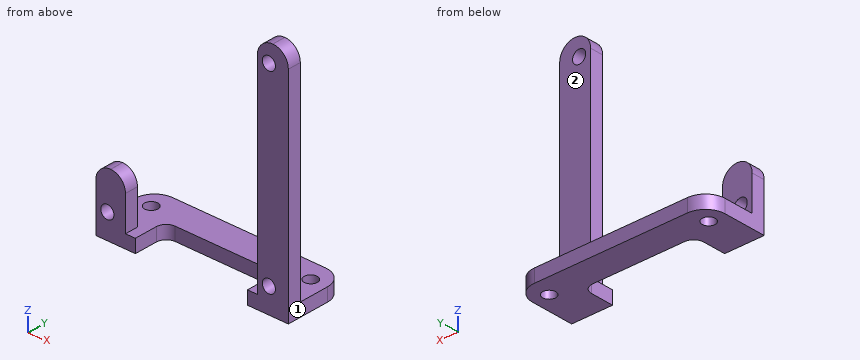
```python
from build123d import *

# Parameters (mm, degrees)
CYLINDER393_R     = 2
CYLINDER393_DEPTH = 16
CYLINDER395_R     = 2
CYLINDER395_DEPTH = 16
CYLINDER394_R     = 2
CYLINDER394_DEPTH = 16
BOX490_W          = 34
BOX490_H          = 10
BOX490_DEPTH      = 7
FILLET028_R       = 3
BOX489_W          = 58.4
BOX489_H          = 19
BOX489_DEPTH      = 4
FILLET029_R       = 6
CYLINDER384_R     = 2
CYLINDER384_DEPTH = 10
CYLINDER385_R     = 2
CYLINDER385_DEPTH = 10
BOX482_W          = 9.4
BOX482_H          = 4
BOX482_DEPTH      = 67
FILLET025_R       = 4.69
CYLINDER386_R     = 2
CYLINDER386_DEPTH = 10
BOX480_W          = 9
BOX480_H          = 4
BOX480_DEPTH      = 15
FILLET024_R       = 4.49


with BuildPart() as cylinder393:
    # Cylinder393 → Cylinder393 (new body)
    with BuildSketch(Plane(origin=(-9.8, 51, -5), x_dir=(1, 0, 0), z_dir=(0, 0, 1))):
        Circle(CYLINDER393_R)
    extrude(amount=CYLINDER393_DEPTH)


with BuildPart() as cylinder395:
    # Cylinder395 → Cylinder395 (new body)
    with BuildSketch(Plane(origin=(-58.2, 51, -5), x_dir=(1, 0, 0), z_dir=(0, 0, 1))):
        Circle(CYLINDER395_R)
    extrude(amount=CYLINDER395_DEPTH)


with BuildPart() as fusion386:
    # Cylinder394 → Cylinder394 (new body)
    with BuildSketch(Plane(origin=(-9.8, 51, -5), x_dir=(1, 0, 0), z_dir=(0, 0, 1))):
        Circle(CYLINDER394_R)
    extrude(amount=CYLINDER394_DEPTH)

    # Fusion386: union Cylinder393, Cylinder395
    add(cylinder393.part)
    add(cylinder395.part)


with BuildPart() as fillet028:
    # Box490 → Box490 (new body)
    with BuildSketch(Plane(origin=(-51.2, 38, 0), x_dir=(1, 0, 0), z_dir=(0, 0, 1))):
        with Locations((17, 5)):
            Rectangle(BOX490_W, BOX490_H)
    extrude(amount=BOX490_DEPTH)

    # Fillet028
    fillet028_edges = [fillet028.edges().sort_by_distance(p)[0] for p in [
        (-51.2, 48, 3.5),
        (-17.2, 48, 3.5),
    ]]
    fillet(fillet028_edges, radius=FILLET028_R)


with BuildPart() as fillet029:
    # Box489 → Box489 (new body)
    with BuildSketch(Plane(origin=(-63.2, 38, 3), x_dir=(1, 0, 0), z_dir=(0, 0, 1))):
        with Locations((29.2, 9.5)):
            Rectangle(BOX489_W, BOX489_H)
    extrude(amount=BOX489_DEPTH)

    # Cut421: cut Fillet028
    add(fillet028.part, mode=Mode.SUBTRACT)

    # Cut422: cut Fusion386
    add(fusion386.part, mode=Mode.SUBTRACT)

    # Fillet029
    fillet029_edges = [fillet029.edges().sort_by_distance(p)[0] for p in [
        (-63.2, 57, 5),
        (-4.8, 57, 5),
    ]]
    fillet(fillet029_edges, radius=FILLET029_R)


with BuildPart() as cylinder384:
    # Cylinder384 → Cylinder384 (new body)
    with BuildSketch(Plane(origin=(-10.7, 44, 10.5), x_dir=(1, 0, 0), z_dir=(0, -1, 0))):
        Circle(CYLINDER384_R)
    extrude(amount=CYLINDER384_DEPTH)


with BuildPart() as fusion379:
    # Cylinder385 → Cylinder385 (new body)
    with BuildSketch(Plane(origin=(-10.7, 44, 68.5), x_dir=(1, 0, 0), z_dir=(0, -1, 0))):
        Circle(CYLINDER385_R)
    extrude(amount=CYLINDER385_DEPTH)

    # Fusion379: union Cylinder384
    add(cylinder384.part)


with BuildPart() as fillet025:
    # Box482 → Box482 (new body)
    with BuildSketch(Plane(origin=(-14.2, 38, 7), x_dir=(1, 0, 0), z_dir=(0, 0, 1))):
        with Locations((4.7, 2)):
            Rectangle(BOX482_W, BOX482_H)
    extrude(amount=BOX482_DEPTH)

    # Cut417: cut Fusion379
    add(fusion379.part, mode=Mode.SUBTRACT)

    # Fillet025
    fillet025_edges = [fillet025.edges().sort_by_distance(p)[0] for p in [
        (-14.2, 40, 74),
        (-4.8, 40, 74),
    ]]
    fillet(fillet025_edges, radius=FILLET025_R)


with BuildPart() as cylinder386:
    # Cylinder386 → Cylinder386 (new body)
    with BuildSketch(Plane(origin=(-59.7, 44, 10.5), x_dir=(1, 0, 0), z_dir=(0, -1, 0))):
        Circle(CYLINDER386_R)
    extrude(amount=CYLINDER386_DEPTH)


with BuildPart() as fusion388:
    # Box480 → Box480 (new body)
    with BuildSketch(Plane(origin=(-63.2, 38, 7), x_dir=(1, 0, 0), z_dir=(0, 0, 1))):
        with Locations((4.5, 2)):
            Rectangle(BOX480_W, BOX480_H)
    extrude(amount=BOX480_DEPTH)

    # Cut418: cut Cylinder386
    add(cylinder386.part, mode=Mode.SUBTRACT)

    # Fillet024
    fillet024_edges = [fusion388.edges().sort_by_distance(p)[0] for p in [
        (-63.2, 40, 22),
        (-54.2, 40, 22),
    ]]
    fillet(fillet024_edges, radius=FILLET024_R)

    # Fusion388: union Fillet029, Fillet025
    add(fillet029.part)
    add(fillet025.part)


solid = fusion388.part
```
The listing builds one solid part. Answer for the finished solid, in the listing's coordinates (mm). Face numbers are marked on the shaded views. A direction names the side the tool comes from. Round coordinates to 2 decimals unless told otherwise and drop trailing zeros. Loops run counter-clockwise (first coordinate to the right, second up) from the corner with the lowest first, then second, coordinate; pieces in that order, holes last. Notation, with made-up numbers: (32, 41.5) - (84, 41.5) arc R19 cw to (84, 64.5) - close; hole circle Ø1 at (57.5, 44). An arc over 180 degrees is marked (long way). Use one line per item in the form item = value. Start each with the question number.
1. The part is cut by section B-B on z = 10.5. Determine the outline of the cut face in (x, y), then the cut area to 3 significant figures.
2. The part is cut by section A-A on y = 43.75. Determine the outline of the cut face in (x, z), then the cut area to 3 significant figures.
3. Consider line 1 (Z direction, x = -10.7, y = 40.85); line 2 (X direction, y = 51, z = 4.2); line 3 (X direction, y = 40.45, z = 68.5). Determine where each line is inside the solid, lowest interval first. Write a range as [from, to].
4. The part is cut by section D-D on x = -29. Determine the outline of the cut face in (y, z), then the cut area to 3 significant figures.
5. A tool of negligible diameter and unlimited length cuts with its end or side. For the marked faces 1 and 2, from which of +Z, -Z, +X, -X, +Y, -Y can it reach the whole face along a straight path? Write none if from no direction.
6. The part is cut by section C-C on z = 68.5. Determine the outline of the cut face in (x, y).
7. Given pin 1 Ø8 at (y, z) = (40, 63.5) entering from -X; pin 2 Ø4.5 at (x, y) = (-58.2, 51) entering from +Z; pin 3 Ø3 at (x, z) = (-40.5, 4.5) entering from -Y, each flat-ended and moving along its own axis, determine where each tip first touches the part or whether it passes through.
Geometry check:
q1.outline = (-63.2, 38) - (-61.7, 38) - (-61.7, 42) - (-63.2, 42) - close; (-57.7, 38) - (-54.2, 38) - (-54.2, 42) - (-57.7, 42) - close; (-14.2, 38) - (-12.7, 38) - (-12.7, 42) - (-14.2, 42) - close; (-8.7, 38) - (-4.8, 38) - (-4.8, 42) - (-8.7, 42) - close
q1.area = 41.6 mm^2
q2.outline = (-63.2, 3) - (-51.2, 3) - (-51.2, 7) - (-63.2, 7) - close; (-17.2, 3) - (-4.8, 3) - (-4.8, 7) - (-17.2, 7) - close
q2.area = 97.6 mm^2
q3.line_1 = [3, 8.5], [12.5, 66.5], [70.5, 73.85]
q3.line_2 = [-63.2, -60.2], [-56.2, -11.8], [-7.8, -4.8]
q3.line_3 = [-14.2, -12.7], [-8.7, -4.8]
q4.outline = (48, 3) - (57, 3) - (57, 7) - (48, 7) - close
q4.area = 36.0 mm^2
q5.face_1 = +Z, -Z, +X, +Y, -Y
q5.face_2 = +Z, +X, -X, +Y
q6.outline = (-14.2, 38) - (-12.7, 38) - (-12.7, 42) - (-14.2, 42) - close; (-8.7, 38) - (-4.8, 38) - (-4.8, 42) - (-8.7, 42) - close
q7.pin_1 = -14.2
q7.pin_2 = 7
q7.pin_3 = 48
